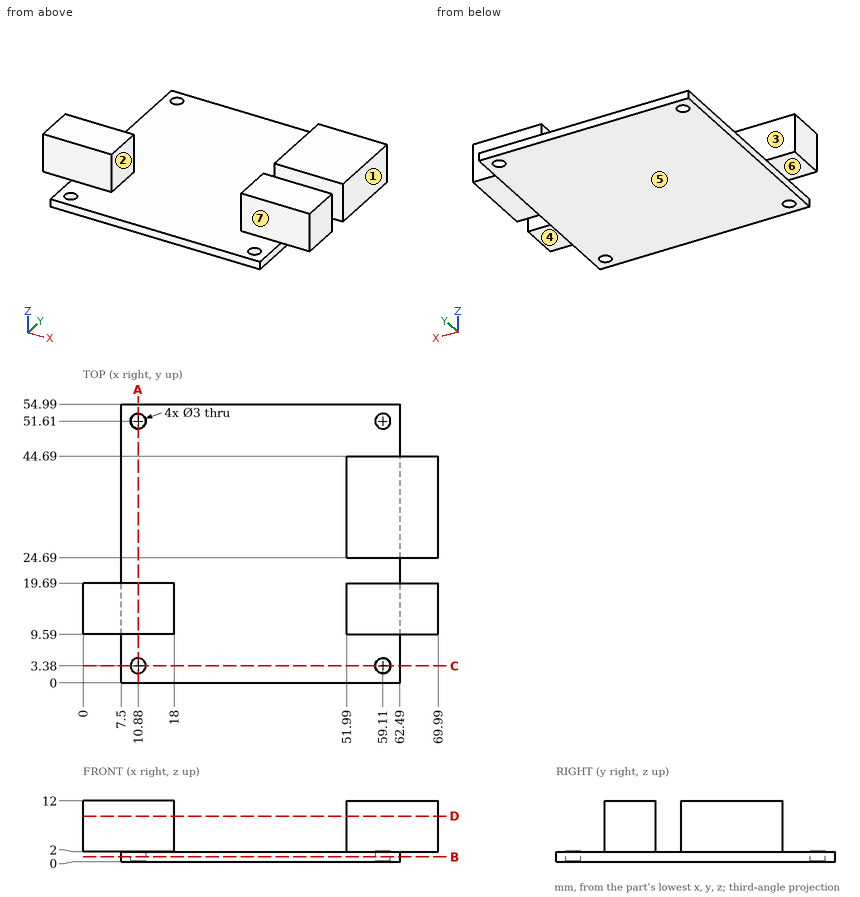
Part print with two shaded views. Sizes in mm from the minimum x, y, z corner. A direction names the side the tool comes from. Round coordinates to 2 decimals unless told otherwise and drop trailing zeros. Order: outer loops, then holes, each group sorted by start corner. A loop starts at its lowest first (then second) coordinate and runs counter-clockwise, first axis right, second up. Notation, with made-up numbers: (42.5, -10.5) -> (68.5, -10.5) arc R25 cw to (68.5, 13.5) -> close; hole circle Ø7 at (50, -22). An arc over 180 degrees is marked (long way). Use one line per item in the form item = value.
Item 1: Tool access for the marked faces 4, 5, 6 and 7: list every direction of +Z, -Z, +X, -X, +Y, -Y with a clear straight run to the whole face (end or side of a thin tool).
Returned:
face_4 = -Z, +X, +Y, -Y
face_5 = -Z, +X, -X, +Y, -Y
face_6 = -Z, -X, +Y, -Y
face_7 = +Z, +X, -X, -Y
Item 2: Cut at B-B, the plane z = 1. Write the cut outline in (x, y), and give its area (3 significant figures).
Returned:
outline = (7.5, 0) -> (62.49, 0) -> (62.49, 54.99) -> (7.5, 54.99) -> close; hole circle Ø3 at (10.88, 3.38); hole circle Ø3 at (10.88, 51.61); hole circle Ø3 at (59.11, 3.38); hole circle Ø3 at (59.11, 51.61)
area = 3,000 mm^2
Item 3: Flat gauge pins, fed straight in: pin 1 Ø1 at (x, y) = (34.5, 10) entering from -Z; pin 2 Ø0.6 at (y, z) = (38, 1) entering from -X; pin 3 Ø5 at (y, z) = (31, 7.5) entering from -X; pin 4 Ø10 at (x, y) = (26.5, 10) entering from +Z. Where does each tip first touch, or does it go through?
Returned:
pin_1 = 0
pin_2 = 7.5
pin_3 = 51.99
pin_4 = 2
Item 4: Drill centre lines: line 1 (Y direction, x = 59.11, z = 0.65); line 2 (X direction, y = 51.61, z = 1.1); line 3 (X direction, y = 17, z = 7). Where is each one in solid material? Low to high.
Returned:
line_1 = 0 to 1.88, 4.88 to 50.11, 53.11 to 54.99
line_2 = 7.5 to 9.38, 12.38 to 57.61, 60.61 to 62.49
line_3 = 0 to 18, 51.99 to 69.99
Item 5: Pull direction X, two halves, no side cores. Call the marked faces 1, 2 and 3: released by +X, released by -X, zero draft, split by the parting line, or undercut.
Returned:
face_1 = released by +X
face_2 = undercut
face_3 = zero draft
Item 6: Cut at A-A, the plane x = 10.88. Write the cut outline in (y, z).
Returned:
outline = (0, 0) -> (1.88, 0) -> (1.88, 2) -> (0, 2) -> close; (4.88, 0) -> (50.11, 0) -> (50.11, 2) -> (19.69, 2) -> (19.69, 12) -> (9.59, 12) -> (9.59, 2) -> (4.88, 2) -> close; (53.11, 0) -> (54.99, 0) -> (54.99, 2) -> (53.11, 2) -> close
Item 7: Cut at C-C, the plane y = 3.38. Write the cut outline in (x, z).
Returned:
outline = (7.5, 0) -> (9.38, 0) -> (9.38, 2) -> (7.5, 2) -> close; (12.38, 0) -> (57.61, 0) -> (57.61, 2) -> (12.38, 2) -> close; (60.61, 0) -> (62.49, 0) -> (62.49, 2) -> (60.61, 2) -> close
Item 8: Cut at D-D, the plane z = 9. Write the cut outline in (x, y), and give its area (3 significant figures).
Returned:
outline = (0, 9.59) -> (18, 9.59) -> (18, 19.69) -> (0, 19.69) -> close; (51.99, 9.59) -> (69.99, 9.59) -> (69.99, 19.69) -> (51.99, 19.69) -> close; (51.99, 24.69) -> (69.99, 24.69) -> (69.99, 44.69) -> (51.99, 44.69) -> close
area = 724 mm^2
